Source: CAD feature listing. Evaluate the final solid. Frame: model axes, mm. A direction names the side the tool comes from. Give positions to 0.01 mm unless a question says otherwise; leave off trailing zeros. Order: outer loops, then holes, each group sorted by start corner. A loop starts at its lowest first (then second) coordinate and runs counter-clockwise, first axis right, second up. Notation, with made-up numbers: (60, 88) - (115, 88) arc R18 ccw to (115, 120) - close; hole circle Ø7 at (57.5, 0.25). An arc over 180 degrees is marked (long way). Use CSV: the item, a comma, the result in double quotes.
```python
from build123d import *

# Parameters (mm, degrees)
F0_W     = 50
F0_H     = 48.4855457247
F1_DEPTH = 10
F2_W     = 30
F2_H     = 8
F4_DEPTH = 40
F3_W     = 30
F3_H     = 8
F5_DEPTH = 40
F7_D     = 5
F8_R     = 14.99999


# Not quite as in the source:
# - a fillet or chamfer is up to 0.001 mm smaller than in the source, because OpenCascade refuses the exact size


with BuildPart() as f1:
    # F0 (on Top) → F1 (new body)
    with BuildSketch(Plane.XY):
        with Locations((-4.2565334588, 1.5670973808)):
            Rectangle(F0_W, F0_H)
    extrude(amount=F1_DEPTH)

    # F2 (on face) → F4 (join)
    with BuildSketch(Plane.XY.offset(10)):
        with Locations((-4.2565334588, 11.8098702431)):
            Rectangle(F2_W, F2_H)
    extrude(amount=F4_DEPTH)

    # F3 (on face) → F5 (join)
    with BuildSketch(Plane.XY.offset(10)):
        with Locations((-4.2565334588, -8.6756754816)):
            Rectangle(F3_W, F3_H)
    extrude(amount=F5_DEPTH)

    # F7 (through all)
    with Locations(Plane.XZ.offset(12.6756754816)):
        with Locations((-4.2565334588, 38)):
            Hole(F7_D / 2)

    # F8 (radius 15 in the source; OpenCascade refuses exactly that, so slightly less here)
    f8_edges = [f1.edges().sort_by_distance(p)[0] for p in [
        (10.743467, -8.675675, 50),
        (-19.256533, -8.675675, 50),
        (10.743467, 11.80987, 50),
        (-19.256533, 11.80987, 50),
    ]]
    fillet(f8_edges, radius=F8_R)


solid = f1.part
```
Item 1: Section D-D on y = -14. Return the cut outline in (x, z).
Filled in:
outline,"(-29.26, 0) - (20.74, 0) - (20.74, 10) - (-29.26, 10) - close"
Item 2: Section A-A on z = 31. Return the cut outline in (x, y), then the cut area to 3 significant figures.
Filled in:
outline,"(-19.26, -12.68) - (10.74, -12.68) - (10.74, -4.68) - (-19.26, -4.68) - close; (-19.26, 7.81) - (10.74, 7.81) - (10.74, 15.81) - (-19.26, 15.81) - close"
area,"480 mm2"
Item 3: First-contact query: pin 1 (15 mm diameter, centred on x = -7.5, z = 38, fed in from -Y); pin 2 (4 mm diameter, centred on y = -7, z = 28.5, fed in from +X); pin 3 (24 mm diameter, centred on x = -6, z = 39.5, fed in from +Y); pin 4 (5 mm diameter, centred on x = -23, z = 40.5, fed in from -Y). Flat tips, straight axial feed; report the tip coordinate or a pass-through.
Filled in:
pin 1,"stops at y = -12.68"
pin 2,"stops at x = 10.74"
pin 3,"stops at y = 15.81"
pin 4,"passes through"
Item 4: Section B-B on x = -11. Return the cut outline in (y, z).
Filled in:
outline,"(-22.68, 0) - (25.81, 0) - (25.81, 10) - (15.81, 10) - (15.81, 48.4) - (7.81, 48.4) - (7.81, 10) - (-4.68, 10) - (-4.68, 48.4) - (-12.68, 48.4) - (-12.68, 10) - (-22.68, 10) - close"
Item 5: Set-up query: faces 1 (the flat face through (10.743, 12, 22)), 2 (the flat face through (-4, -12.676, 30)), 3 (the flat face through (-19.257, -9, 22)). Return all of +Z, -Z, +X, -X, +Y, -Y with unobstructed straight access to the full face (end or side cutting, diameter ignored); none if empty.
Filled in:
face 1,"+Z, +X, +Y, -Y"
face 2,"+Z, +X, -X, -Y"
face 3,"+Z, -X, +Y, -Y"
Item 6: Section C-C on z = 38. Return the cut outline in (x, y), then the cut area to 3 significant figures.
Filled in:
outline,"(-18.95, -12.68) - (-6.76, -12.68) - (-6.76, -4.68) - (-18.95, -4.68) - close; (-18.95, 7.81) - (-6.76, 7.81) - (-6.76, 15.81) - (-18.95, 15.81) - close; (-1.76, -12.68) - (10.44, -12.68) - (10.44, -4.68) - (-1.76, -4.68) - close; (-1.76, 7.81) - (10.44, 7.81) - (10.44, 15.81) - (-1.76, 15.81) - close"
area,"390 mm2"
Item 7: Material intervals for line 1 (Y direction, x = 5, z = 39); line 2 (X direction, y = 9, z = 15); line 3 (X direction, y = 12, z = 36.5), sorted ascending. Write a range as from..to.
Filled in:
line 1,"y = -12.68..-4.68, 7.81..15.81"
line 2,"x = -19.26..10.74"
line 3,"x = -19.18..-6.26, -2.26..10.67"
Item 8: Mould query, pull axis Y, two halves, no side actions, for faces 4 (the flat face through (-5, 2, 10)), 5 (the flat face through (-5, 2, 0)), 6 (the flat face through (-5, -22.676, 5)). Classes: released by +Y, released by -Y, zero draft, split by the parting line, or undercut.
Filled in:
face 4,"undercut"
face 5,"zero draft"
face 6,"released by -Y"
